Study the drawing (mm; zero at the part's minimum x, y, z) and answer. A direction names the side the tool comes from. Give positions to 0.01 mm unless a question says otherwise; leave off trailing zeros. Order: outer loops, then holes, each group sorted by start corner. A loop starts at its lowest first (then second) coordinate and runs counter-clockwise, first axis right, second up. Notation, with made-up numbers: (-29, -19) - (-17, -19) arc R31 ccw to (-17, 7) - close; hole circle Ø9 at (-31.5, 67.5). An arc over 180 degrees is marked (long way). Put each result on its own line as item: value.
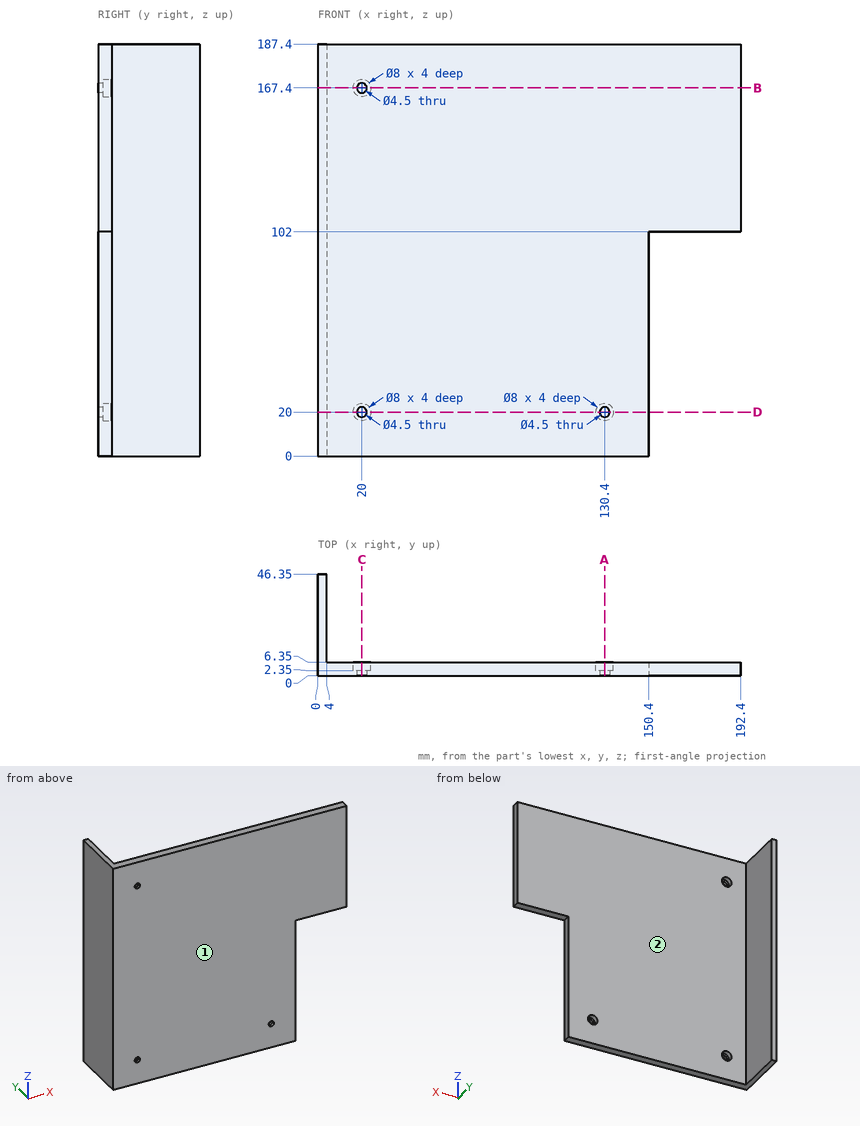
(1) A tool of negligible diameter and unlimited length cuts with its end or side. For the marked faces 1 and 2, from which of +Z, -Z, +X, -X, +Y, -Y can it reach the whole face along a straight path? Write none if from no direction.
Geometry check:
face 1: +Z, -Z, +X, -X, -Y
face 2: +Z, -Z, +X, +Y
(2) Straight lines are drawn through the part: line 1 (X direction, y = 3.3, z = 20); line 2 (Z direction, x = 20, y = 1); line 3 (Z direction, x = 20, y = 5). For each, find the intervals that lie inside material, in ascending order.
Geometry check:
line 1: x = 0 to 16, 24 to 126.4, 134.4 to 150.4
line 2: z = 0 to 17.75, 22.25 to 165.15, 169.65 to 187.4
line 3: z = 0 to 16, 24 to 163.4, 171.4 to 187.4
(3) Section B-B, the plane z = 167.4 is taken. Write down the section's boundary in (x, y).
Geometry check:
outline: (0, 0) - (17.75, 0) - (17.75, 2.35) - (16, 2.35) - (16, 6.35) - (4, 6.35) - (4, 46.35) - (0, 46.35) - close; (22.25, 0) - (192.4, 0) - (192.4, 6.35) - (24, 6.35) - (24, 2.35) - (22.25, 2.35) - close
(4) Given pin 1 (9 mm diameter, centred on x = 130, z = 21, fed in from +Y); pin 2 (7 mm diameter, centred on x = 173, y = 3, fed in from -Z); pin 3 (7 mm diameter, centred on y = 4.5, z = 40, fed in from +X); pin 4 (5 mm diameter, centred on x = 130.4, z = 20, fed in from -Y), each flat-ended and moving along its own axis, determine where each tip first touches the part or whether it passes through.
Geometry check:
pin 1: stops at y = 6.35
pin 2: stops at z = 102
pin 3: stops at x = 150.4
pin 4: stops at y = 0
(5) Section A-A, the plane x = 130.4 is taken. Write down the section's boundary in (y, z), then the cut area to 3 significant figures.
Geometry check:
outline: (0, 0) - (6.35, 0) - (6.35, 16) - (2.35, 16) - (2.35, 17.75) - (0, 17.75) - close; (0, 22.25) - (2.35, 22.25) - (2.35, 24) - (6.35, 24) - (6.35, 187.4) - (0, 187.4) - close
area: 1,150 mm²
(6) Section D-D, the plane z = 20 is taken. Write down the section's boundary in (x, y), then the cut area to 3 significant figures.
Geometry check:
outline: (0, 0) - (17.75, 0) - (17.75, 2.35) - (16, 2.35) - (16, 6.35) - (4, 6.35) - (4, 46.35) - (0, 46.35) - close; (22.25, 0) - (128.15, 0) - (128.15, 2.35) - (126.4, 2.35) - (126.4, 6.35) - (24, 6.35) - (24, 2.35) - (22.25, 2.35) - close; (132.65, 0) - (150.4, 0) - (150.4, 6.35) - (134.4, 6.35) - (134.4, 2.35) - (132.65, 2.35) - close
area: 1,030 mm²
(7) Section C-C, the plane x = 20 is taken. Write down the section's boundary in (y, z).
Geometry check:
outline: (0, 0) - (6.35, 0) - (6.35, 16) - (2.35, 16) - (2.35, 17.75) - (0, 17.75) - close; (0, 22.25) - (2.35, 22.25) - (2.35, 24) - (6.35, 24) - (6.35, 163.4) - (2.35, 163.4) - (2.35, 165.15) - (0, 165.15) - close; (0, 169.65) - (2.35, 169.65) - (2.35, 171.4) - (6.35, 171.4) - (6.35, 187.4) - (0, 187.4) - close
